from build123d import *

# Parameters (mm, degrees)
BOSS_EXTRUDE1_DEPTH = 5.842
SKETCH2_W           = 5.460302537
SKETCH2_H           = 25.4
CUT_EXTRUDE1_DEPTH  = 48.288535112
FILLET2_R           = 1.5875


with BuildPart() as part:
    # Sketch1 → Boss-Extrude1 (new body)
    with BuildSketch(Plane(origin=(0, 0, 0), x_dir=(1, 0, 0), z_dir=(0, 1, 0))):
        Polygon((-6.45, 31.342), (-6.45, 25.5), (-11.335313542, 25.5), (-11.335313542, 19.15), (-8.73125, 19.15), (-8.73125, 16.371875), (-11.286067573, 16.371875), (-11.286067573, 11.892), (-14.113932427, 11.892), (-14.113932427, 16.371875), (-16.66875, 16.371875), (-16.66875, 19.15), (-14.064686458, 19.15), (-14.064686458, 25.5), (-18.95, 25.5), (-18.95, 31.342), (-31.85, 31.342), (-31.85, 25.5), (-34.925, 25.5), (-34.925, -25.5), (-31.85, -25.5), (-31.85, -31.342), (-18.95, -31.342), (-18.95, -25.5), (-14.064686458, -25.5), (-14.064686458, -19.15), (-16.66875, -19.15), (-16.66875, -16.371875), (-14.113932427, -16.371875), (-14.113932427, -11.892), (-11.286067573, -11.892), (-11.286067573, -16.371875), (-8.73125, -16.371875), (-8.73125, -19.15), (-11.335313542, -19.15), (-11.335313542, -25.5), (-6.45, -25.5), (-6.45, -31.342), (6.45, -31.342), (6.45, -25.5), (11.335313542, -25.5), (11.335313542, -19.15), (8.73125, -19.15), (8.73125, -16.371875), (11.286067573, -16.371875), (11.286067573, -11.892), (14.113932427, -11.892), (14.113932427, -16.371875), (16.66875, -16.371875), (16.66875, -19.15), (14.064686458, -19.15), (14.064686458, -25.5), (18.95, -25.5), (18.95, -31.342), (31.85, -31.342), (31.85, -25.5), (34.925, -25.5), (34.925, 25.5), (31.85, 25.5), (31.85, 31.342), (18.95, 31.342), (18.95, 25.5), (14.064686458, 25.5), (14.064686458, 19.15), (16.66875, 19.15), (16.66875, 16.371875), (14.113932427, 16.371875), (14.113932427, 11.892), (11.286067573, 11.892), (11.286067573, 16.371875), (8.73125, 16.371875), (8.73125, 19.15), (11.335313542, 19.15), (11.335313542, 25.5), (6.45, 25.5), (6.45, 31.342), align=None)
    extrude(amount=BOSS_EXTRUDE1_DEPTH)

    # Sketch2 → Cut-Extrude1 (cut, through all)
    with BuildSketch(Plane(origin=(0, 5.842, 0), x_dir=(1, 0, 0), z_dir=(0, 1, 0))):
        with Locations((-32.194848732, 0)):
            Rectangle(SKETCH2_W, SKETCH2_H)
        with Locations((32.194848732, 0)):
            Rectangle(SKETCH2_W, SKETCH2_H)
    extrude(amount=-CUT_EXTRUDE1_DEPTH, mode=Mode.SUBTRACT)

    # Fillet2
    fillet2_edges = [part.edges().sort_by_distance(p)[0] for p in [
        (-34.925, 2.921, -12.7),
        (-29.464697463, 2.921, -12.7),
        (-29.464697463, 2.921, 12.7),
        (-34.925, 2.921, 12.7),
        (29.464697463, 2.921, -12.7),
        (34.925, 2.921, -12.7),
        (34.925, 2.921, 12.7),
        (29.464697463, 2.921, 12.7),
    ]]
    fillet(fillet2_edges, radius=FILLET2_R)


solid = part.part
Part model, mm, in its own coordinate system. A direction names the side the tool comes from. Give positions to 0.01 mm unless a question says otherwise; leave off trailing zeros. Write each loop counter-clockwise with the first axis right and the second up, starting at its lowest first coordinate (ties: lowest second). Pieces come first, ordered by that corner, then holes.
1) Cut at C-C on z = -8. Write the cut outline in (x, y).
Resolved:
outline: (-29.46, 0) - (29.46, 0) - (29.46, 5.84) - (-29.46, 5.84) - close
2) Pin check, flat tips, straight feed: pin 1 (3.5 mm diameter, centred on y = 4, z = 14, fed in from +X) (3 decimals); pin 2 (3 mm diameter, centred on y = 3.5, z = 29.5, fed in from -X); pin 3 (1.4 mm diameter, centred on x = -13, y = 2, fed in from +Z); pin 4 (0.8 mm diameter, centred on x = 15, y = 3, fed in from +Z). Stop position of each tip, or through.
Resolved:
pin 1: stops at x = 34.925
pin 2: stops at x = -31.85
pin 3: stops at z = 11.89
pin 4: stops at z = 25.5
3) Which spindle directions (+Z, -Z, +X, -X, +Y, -Y) get a long thin tool onto all of the face, cutting with end or side? Do faces 1 (the face through (-34.472, 2.88, 13.177)), 2 (the face through (-33, 3, 25.5)), 3 (the face through (-8.731, 3, -18)), 4 (the face through (11.335, 3, 22)). Say none if no direction does.
Resolved:
face 1: -X, +Y, -Y
face 2: +Z, -X, +Y, -Y
face 3: +Y, -Y
face 4: +Z, +Y, -Y
4) Cut at B-B on z = 17.5. Write the cut outline in (x, y) (3 decimals), then the cut area to 3 significant figures.
Resolved:
outline: (-34.925, 0) - (-16.669, 0) - (-16.669, 5.842) - (-34.925, 5.842) - close; (-8.731, 0) - (8.731, 0) - (8.731, 5.842) - (-8.731, 5.842) - close; (16.669, 0) - (34.925, 0) - (34.925, 5.842) - (16.669, 5.842) - close
area: 315 mm2
5) Two-plate mould, pull along Z, no slides. Class faces 5 (the face through (34.448, 2.88, 13.153)), 6 (the face through (-8.731, 3, 18)), 7 (the face through (-17, 3, 25.5)): released by +Z, released by -Z, zero draft, split by the parting line, or undercut.
Resolved:
face 5: undercut
face 6: undercut
face 7: released by +Z
6) Cut at A-A on x = -15. Write the cut outline in (y, z).
Resolved:
outline: (0, -25.5) - (5.84, -25.5) - (5.84, -19.15) - (0, -19.15) - close; (0, -16.37) - (5.84, -16.37) - (5.84, 16.37) - (0, 16.37) - close; (0, 19.15) - (5.84, 19.15) - (5.84, 25.5) - (0, 25.5) - close
7) Probe L1, parallel to Z at x = 15.5, y = 4.95; L2, parallel to X at y = 3.3, z = 15 (3 decimals); L3, parallel to X at y = 1, z = 18.5 (3 decimals). List the from-to ranges inside material, lowest first.
Resolved:
L1: z = -25.5 to -19.15, -16.37 to 16.37, 19.15 to 25.5
L2: x = -34.925 to -14.114, -11.286 to 11.286, 14.114 to 34.925
L3: x = -34.925 to -16.669, -8.731 to 8.731, 16.669 to 34.925
